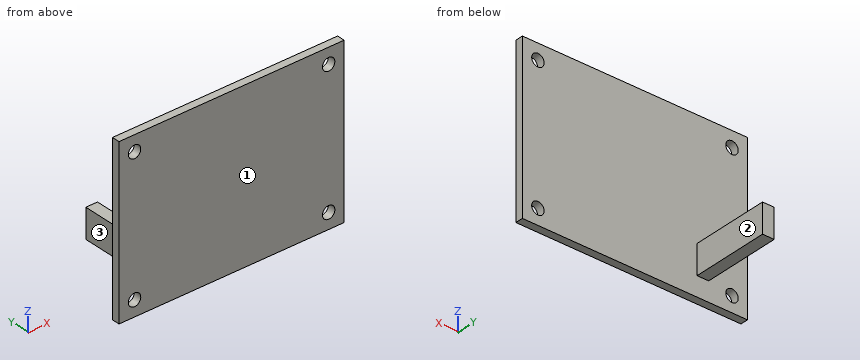
```python
from build123d import *

# Parameters (mm, degrees)
SKETCH_1_W          = 58
SKETCH_1_H          = 42.5
EXTRUDE_1_DEPTH     = 2
SKETCH_2_R          = 1.6
CUT_EXTRUDE_1_DEPTH = 3
SKETCH_3_W          = 3
SKETCH_3_H          = 7.5
EXTRUDE_2_DEPTH     = 20


with BuildPart() as part:
    # 草图1 → 凸台-拉伸1 (new body)
    with BuildSketch(Plane(origin=(0, 0, 0), x_dir=(1, 0, 0), z_dir=(0, 1, 0))):
        with Locations((29, 21.25)):
            Rectangle(SKETCH_1_W, SKETCH_1_H)
    extrude(amount=EXTRUDE_1_DEPTH)

    # 草图2 → 切除-拉伸1 (cut, through all)
    with BuildSketch(Plane(origin=(0, 2, 0), x_dir=(1, 0, 0), z_dir=(0, 1, 0))):
        with Locations((54, 38.5)):
            Circle(SKETCH_2_R)
        with Locations((54, 4)):
            Circle(SKETCH_2_R)
        with Locations((4, 4)):
            Circle(SKETCH_2_R)
        with Locations((4, 38.5)):
            Circle(SKETCH_2_R)
    extrude(amount=-CUT_EXTRUDE_1_DEPTH, mode=Mode.SUBTRACT)

    # 草图3 → 凸台-拉伸2 (add)
    with BuildSketch(Plane(origin=(0, 2, 0), x_dir=(1, 0, 0), z_dir=(0, 1, 0))):
        with Locations((11.5, 33.75)):
            Rectangle(SKETCH_3_W, SKETCH_3_H)
    extrude(amount=EXTRUDE_2_DEPTH)


solid = part.part
```
Design review of the part built by this model. Coordinates are the model's own, in mm. Face numbers are marked on the shaded views. A direction names the side the tool comes from. Coordinates: 2 decimals unless noted, no trailing zeros. Order: outer loops, then holes, each group sorted by start corner. A loop starts at its lowest first (then second) coordinate and runs counter-clockwise, first axis right, second up. Notation, with made-up numbers: (1.5, -38) - (50.5, -38) arc R19 ccw to (50.5, -13) - close; hole circle Ø7 at (7, 41.25). An arc over 180 degrees is marked (long way). Answer in a Markdown table with one row per item.
(1) For the marked faces 1, 2 and 3, list the 3-axis set-ups (+Z, -Z, +X, -X, +Y, -Y) from which the entire face can be reached by the end or side of a thin tool; tool diameter is ignored.
Checked values:
| item | result |
|---|---|
| face 1 | +Z, -Z, +X, -X, -Y |
| face 2 | +Z, -Z, +X, +Y |
| face 3 | +Z, -Z, -X, +Y |
(2) Wall thickness on line 1 along X through (y, z) = (0.65, -4); line 2 along Z through (x, y) = (54, 1.2); line 3 along Y through (x, z) = (30, -29): over which ranges is each line inside the solid? List them lowest first. Write a range as from..to.
Checked values:
| item | result |
|---|---|
| line 1 | 0..2.4, 5.6..52.4, 55.6..58 |
| line 2 | -42.5..-40.1, -36.9..-5.6, -2.4..0 |
| line 3 | 0..2 |
(3) Consider section D-D on y = 15.25. State the section outline as (x, z) points, plus the area to 3 significant figures.
Checked values:
| item | result |
|---|---|
| outline | (10, -37.5) - (13, -37.5) - (13, -30) - (10, -30) - close |
| area | 22.5 mm^2 |
(4) Clearance check with flat-ended pins moving along their axes: pin 1 (4 mm diameter, centred on x = 25.5, z = -11.5, fed in from +Y); pin 2 (3.5 mm diameter, centred on x = 11, y = 9, fed in from -Z); pin 3 (2 mm diameter, centred on y = 16, z = -34.5, fed in from +X); pin 4 (2.5 mm diameter, centred on x = 4, z = -4, fed in from +Y). State where each tip first meets the part, or that it passes through.
Checked values:
| item | result |
|---|---|
| pin 1 | y = 2 |
| pin 2 | z = -37.5 |
| pin 3 | x = 13 |
| pin 4 | through |
(5) Consider section B-B on z = -4. State the section outline as (x, y) points, plus the area to 3 significant figures.
Checked values:
| item | result |
|---|---|
| outline | (0, 0) - (2.4, 0) - (2.4, 2) - (0, 2) - close; (5.6, 0) - (52.4, 0) - (52.4, 2) - (5.6, 2) - close; (55.6, 0) - (58, 0) - (58, 2) - (55.6, 2) - close |
| area | 103 mm^2 |
(6) Consider section A-A on x = 54. State the section outline as (y, z) points.
Checked values:
| item | result |
|---|---|
| outline | (0, -42.5) - (2, -42.5) - (2, -40.1) - (0, -40.1) - close; (0, -36.9) - (2, -36.9) - (2, -5.6) - (0, -5.6) - close; (0, -2.4) - (2, -2.4) - (2, 0) - (0, 0) - close |
(7) Consider section C-C on z = -31. State the section outline as (x, y) points, plus the area to 3 significant figures.
Checked values:
| item | result |
|---|---|
| outline | (0, 0) - (58, 0) - (58, 2) - (13, 2) - (13, 22) - (10, 22) - (10, 2) - (0, 2) - close |
| area | 176 mm^2 |
